Verification items for the finished model (mm, model axes). Face numbers are marked on the shaded views. A direction names the side the tool comes from. Give positions to 0.01 mm unless a question says otherwise; leave off trailing zeros. Order: outer loops, then holes, each group sorted by start corner. A loop starts at its lowest first (then second) coordinate and runs counter-clockwise, first axis right, second up. Notation, with made-up numbers: M 69,61.5 L 105,61.5 A23 ccw 105,97.5 Z; hole C 65.5,87.5 d10. An arc over 180 degrees is marked long. Answer as a JSON object with one key per item and string values.
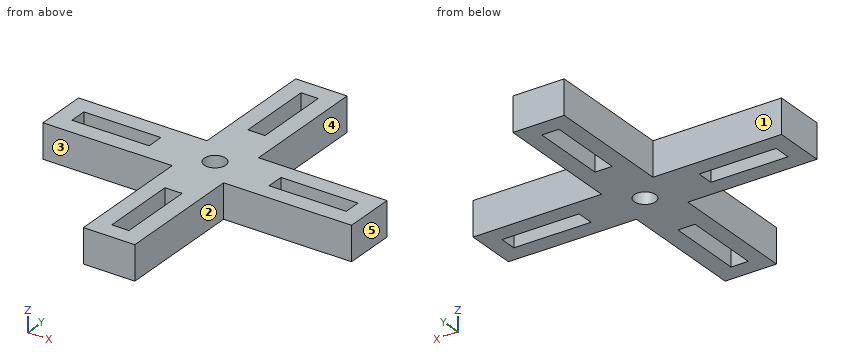
```python
from build123d import *

# Parameters (mm, degrees)
ESQUISSE1_W             = 2
ESQUISSE1_H             = 9
ESQUISSE1_W_2           = 9
ESQUISSE1_H_2           = 2
BOSS_EXTRU_4_DEPTH      = 4
ESQUISSE2_R             = 1.25
ENL_V_MAT_EXTRU_1_DEPTH = 4


with BuildPart() as part:
    # Esquisse1 → Boss.-Extru.4 (new body)
    with BuildSketch(Plane.XY):
        Polygon((0, 0), (-6, 0), (-6, -15), (-21, -15), (-21, -21), (-5.927854654, -21), (-5.927854654, -36), (0.072145346, -36), (0.072145346, -21), (15, -21), (15, -15), (0, -15), align=None)
        with Locations((-3, -6.5)):
            Rectangle(ESQUISSE1_W, ESQUISSE1_H, mode=Mode.SUBTRACT)
        with Locations((-14.5, -18)):
            Rectangle(ESQUISSE1_W_2, ESQUISSE1_H_2, mode=Mode.SUBTRACT)
        with Locations((-3, -29.5)):
            Rectangle(ESQUISSE1_W, ESQUISSE1_H, mode=Mode.SUBTRACT)
        with Locations((8.5, -18)):
            Rectangle(ESQUISSE1_W_2, ESQUISSE1_H_2, mode=Mode.SUBTRACT)
    extrude(amount=BOSS_EXTRU_4_DEPTH)

    # Esquisse2 → Enlèv. mat.-Extru.1 (cut)
    with BuildSketch(Plane.XY.offset(4)):
        with Locations((-3, -18)):
            Circle(ESQUISSE2_R)
    extrude(amount=-ENL_V_MAT_EXTRU_1_DEPTH, mode=Mode.SUBTRACT)


solid = part.part
```
Q1. Section check C-C on z = 1.1. Count the separate pieces of the cut face and the enclosed holes in it, then the cut area to 3 significant figures.
Resolved:
{"separate pieces": "1", "enclosed holes": "5", "area": "319 mm²"}
Q2. Material ranges on L1, parallel to Y at x = -3, z = 2; L2, parallel to Y at x = -17, z = 0.8; L3, parallel to X at y = -25.5, z = 2.75, recorded low to high.
Resolved:
{"L1": "y = -36 to -34, -25 to -19.25, -16.75 to -11, -2 to 0", "L2": "y = -21 to -19, -17 to -15", "L3": "x = -5.93 to -4, -2 to 0.07"}
Q3. Tool access check on the marked faces 1, 2, 3, 4 and 5. Record the directions out of +Z, -Z, +X, -X, +Y, -Y that give a thin tool (end or side, any length) a straight path to the whole face; none if there is none.
Resolved:
{"face 1": "+Z, -Z, -X, +Y", "face 2": "+Z, -Z, +X, -Y", "face 3": "+Z, -Z, -X, -Y", "face 4": "+Z, -Z, +X, +Y", "face 5": "+Z, -Z, +X, +Y, -Y"}
Q4. Section check D-D on x = 5.5. Record the cut outline in (y, z), then the cut area to 3 significant figures.
Resolved:
{"outline": "M -21,0 L -19,0 L -19,4 L -21,4 Z; M -17,0 L -15,0 L -15,4 L -17,4 Z", "area": "16.0 mm²"}
Q5. Gauge pin test, flat ends, axial feed: pin 1 Ø1.2 at (x, z) = (10, 1) entering from +Y; pin 2 Ø5 at (x, y) = (1, -21) entering from -Z; pin 3 Ø2 at (x, z) = (-13.5, 1) entering from -Y; pin 4 Ø1.2 at (y, z) = (-8, 2.5) entering from -X. Record the tip position at first contact, or that the pin passes through.
Resolved:
{"pin 1": "stops at y = -15", "pin 2": "stops at z = 0", "pin 3": "stops at y = -21", "pin 4": "stops at x = -6"}
Q6. Section check B-B on y = -18. Record the cut outline in (x, z), then the cut area to 3 significant figures.
Resolved:
{"outline": "M -21,0 L -19,0 L -19,4 L -21,4 Z; M -10,0 L -4.25,0 L -4.25,4 L -10,4 Z; M -1.75,0 L 4,0 L 4,4 L -1.75,4 Z; M 13,0 L 15,0 L 15,4 L 13,4 Z", "area": "62.0 mm²"}
Q7. Section check A-A on x = -3. Record the cut outline in (y, z).
Resolved:
{"outline": "M -36,0 L -34,0 L -34,4 L -36,4 Z; M -25,0 L -19.25,0 L -19.25,4 L -25,4 Z; M -16.75,0 L -11,0 L -11,4 L -16.75,4 Z; M -2,0 L 0,0 L 0,4 L -2,4 Z"}
